Verification items for the finished model (mm, model axes). Coordinates: 2 decimals unless noted, no trailing zeros. Write each loop counter-clockwise with the first axis right and the second up, starting at its lowest first coordinate (ties: lowest second). Pieces come first, ordered by that corner, then holes. Notation, with made-up numbers: (-28.75, 17.25) -> (21.25, 17.25) arc R31 cw to (21.25, 43.25) -> close; hole circle Ø3 at (4.5, 60). An arc over 180 degrees is marked (long way). Answer in a Markdown table with one row per item.
```python
from build123d import *

# Parameters (mm, degrees)
SKETCH1_R          = 15.875
BASE_EXTRUDE_DEPTH = 3.175


with BuildPart() as part:
    # Sketch1 → Base-Extrude (new body)
    with BuildSketch(Plane.XY):
        with BuildLine():
            Line((-725.551, -96.926304331), (-652.5006, -360.027421394))
            ThreePointArc((-652.5006, -360.027421394), (0, -273.05), (652.5006, -360.027421394))
            Line((652.5006, -360.027421394), (725.551, -96.926304331))
            ThreePointArc((725.551, -96.926304331), (0, 0), (-725.551, -96.926304331))
        make_face()
        with Locations((0, -80.7212)):
            Circle(SKETCH1_R, mode=Mode.SUBTRACT)
        with Locations((-50.8, -80.7212)):
            Circle(SKETCH1_R, mode=Mode.SUBTRACT)
        with Locations((-101.6, -80.7212)):
            Circle(SKETCH1_R, mode=Mode.SUBTRACT)
        with Locations((50.8, -80.7212)):
            Circle(SKETCH1_R, mode=Mode.SUBTRACT)
        with Locations((101.6, -80.7212)):
            Circle(SKETCH1_R, mode=Mode.SUBTRACT)
    extrude(amount=-BASE_EXTRUDE_DEPTH)


solid = part.part
```
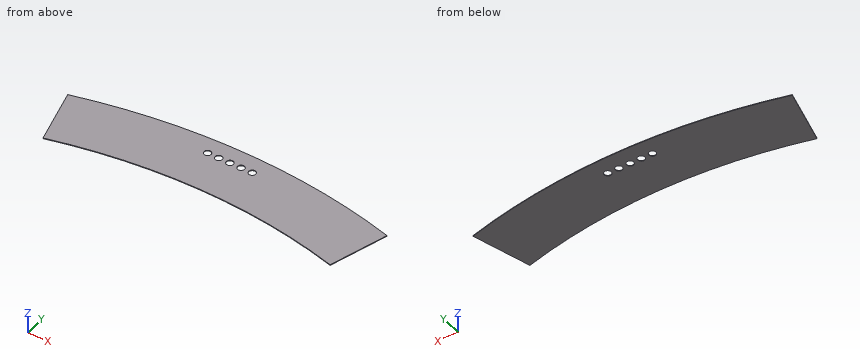
1. Sectioned sample at D-D, the plane x = 417.5. Record the cut outline in (y, z) (3 decimals), and give its area (3 significant figures).
Findings below:
| item | result |
|---|---|
| outline | (-308.286, -3.175) -> (-31.713, -3.175) -> (-31.713, 0) -> (-308.286, 0) -> close |
| area | 878 mm² |
2. Sectioned sample at B-B, the plane z = -2.05. Record the cut outline in (x, y) (3 decimals).
Findings below:
| item | result |
|---|---|
| outline | (-725.551, -96.926) -> (-652.501, -360.027) arc R2491.003 cw to (652.501, -360.027) -> (725.551, -96.926) arc R2764.053 ccw to start; hole circle Ø31.75 at (-101.6, -80.721); hole circle Ø31.75 at (-50.8, -80.721); hole circle Ø31.75 at (0, -80.721); hole circle Ø31.75 at (50.8, -80.721); hole circle Ø31.75 at (101.6, -80.721) |
3. Sectioned sample at C-C, the plane x = -200.5. Record the cut outline in (y, z) (3 decimals).
Findings below:
| item | result |
|---|---|
| outline | (-281.132, -3.175) -> (-7.282, -3.175) -> (-7.282, 0) -> (-281.132, 0) -> close |
4. Material ranges on probe 1 along Y at (x, z) = (-9.5, -1.8); probe 2 along Y at (x, z) = (50.8, -1.3); probe 3 along Y at (x, z) = (301, -0.6), recorded low to high. Write a range as from..to.
Findings below:
| item | result |
|---|---|
| probe 1 | y = -273.07..-93.44, -68..-0.02 |
| probe 2 | y = -273.57..-96.6, -64.85..-0.47 |
| probe 3 | y = -291.3..-16.44 |
5. Sectioned sample at A-A, the plane x = 0. Record the cut outline in (y, z) (3 decimals).
Findings below:
| item | result |
|---|---|
| outline | (-273.05, -3.175) -> (-96.596, -3.175) -> (-96.596, 0) -> (-273.05, 0) -> close; (-64.846, -3.175) -> (0, -3.175) -> (0, 0) -> (-64.846, 0) -> close |
